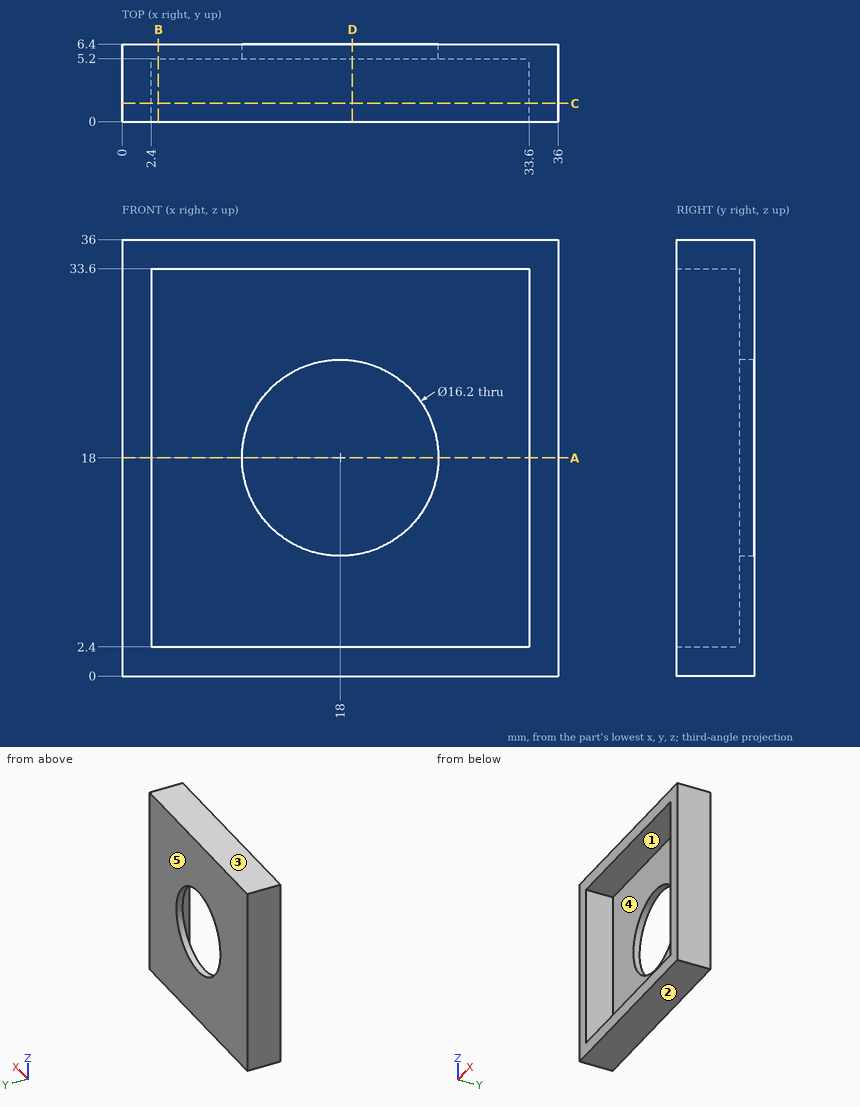
Answer from the drawing. Dimensions are ordinates in mm from the lowest x, y and z of the part. A direction names the side the tool comes from. Round coordinates to 2 decimals unless told otherwise and drop trailing zeros. Write each loop counter-clockwise with the first axis right and the second up, starting at its lowest first coordinate (ties: lowest second). Pieces come first, ordered by that corner, then holes.
1. Determine the mould class of the marked faces 3, 4 and 5 for opening direction Z: pulls with the +Z half, pulls with the -Z half, needs draft (parallel to the pull), parting line crosses it, or undercut.
2. The part is cut by section B-B, the plane x = 3. Determine the outline of the cut face in (y, z).
3. The part is cut by section D-D, the plane x = 19. Determine the outline of the cut face in (y, z), then the cut area to 3 significant figures.
4. Straight lines are drawn through the part: L1, parallel to X at y = 2, z = 21; L2, parallel to X at y = 5.95, z = 18. For each, find the intervals that lie inside material, in ascending order.
5. Which of the six approach directions +Z, -Z, +X, -X, +Y, -Y give full straight-line access (tool end or side, diameter ignored) to the marked faces 1 and 2?
6. The part is cut by section C-C, the plane y = 1.5. Determine the outline of the cut face in (x, z).
7. The part is cut by section A-A, the plane z = 18. Determine the outline of the cut face in (x, y).
8. Given pin 1 Ø21 at (x, z) = (18, 18) entering from -Y, flat-ended and moving along its own axis, determine where the tip first touches the part or whether it passes through.
Values:
1. face 3: pulls with the +Z half
1. face 4: undercut
1. face 5: needs draft
2. outline: (0, 0) - (6.4, 0) - (6.4, 36) - (0, 36) - (0, 33.6) - (5.2, 33.6) - (5.2, 2.4) - (0, 2.4) - close
3. outline: (0, 0) - (6.4, 0) - (6.4, 9.96) - (5.2, 9.96) - (5.2, 2.4) - (0, 2.4) - close; (0, 33.6) - (5.2, 33.6) - (5.2, 26.04) - (6.4, 26.04) - (6.4, 36) - (0, 36) - close
3. area: 48.9 mm2
4. L1: x = 0 to 2.4, 33.6 to 36
4. L2: x = 0 to 9.9, 26.1 to 36
5. face 1: -Y
5. face 2: -Z, +X, -X, +Y, -Y
6. outline: (0, 0) - (36, 0) - (36, 36) - (0, 36) - close; hole (2.4, 2.4) - (33.6, 2.4) - (33.6, 33.6) - (2.4, 33.6) - close
7. outline: (0, 0) - (2.4, 0) - (2.4, 5.2) - (9.9, 5.2) - (9.9, 6.4) - (0, 6.4) - close; (26.1, 5.2) - (33.6, 5.2) - (33.6, 0) - (36, 0) - (36, 6.4) - (26.1, 6.4) - close
8. pin 1: stops at y = 5.2
